Source: CAD feature listing. Evaluate the final solid. Frame: model axes, mm. A direction names the side the tool comes from. Round coordinates to 2 decimals unless told otherwise and drop trailing zeros. Write each loop counter-clockwise with the first axis right and the second up, starting at its lowest first coordinate (ties: lowest second). Pieces come first, ordered by that corner, then holes. Notation, with made-up numbers: M -11,41 L 41,41 A25 cw 41,57 Z; hole C 81,80.5 d9. An arc over 180 degrees is marked long. Answer in a Markdown table with one row per item.
Autodesk Inventor part; units mm, degrees
ref_plane "Work Plane1" through (1.525, 0, 0) normal (0, 0, 1) x (1, 0, 0)
ref_plane "YZ Plane" through (0, 0, 0) normal (1, 0, 0) x (0, 1, 0)
ref_plane "XZ Plane" through (0, 0, 0) normal (0, 1, 0) x (-1, 0, 0)
sketch "草图1" plane through (0, 0, 0) normal (0, 0, 1) x (1, 0, 0)
  line L0 (0, 5.8) -> (0, 4)
  line L1 (1.25, 4) -> (25, 4)
  line L2 (25, 4) -> (25, 0)
  line L3 (25, 0) -> (-0.6001, 0)
  line L4 (-5.7201, 0) -> (30.12, 0)
  line L5 (-0.6001, 0) -> (-0.6001, 5.8)
  line L6 (-0.6001, 5.8) -> (0, 5.8)
  line L7 (1.25, 4) -> (0.4831, 4)
  line L8 (0.4831, 4) -> (0, 4)
  line L9 (0, -1.16) -> (0, 6.96)
  dimension "d0" = 25
  dimension "d1" = 23.75
  dimension "d2" = 8
  dimension "d9" = 0.6001
  dimension "d10" = 11.6
  dimension "d13" = 0.7669
  dimension "d14" = 8
revolve "轴承体" add sketch "草图1" angle 360 about axis through (25, 0, 0) along (-1, 0, 0)
sketch "草图2" plane through (-0.6001, 0, 0) normal (-1, 0, 0) x (0, 0, 1)
  line L0 (0, 7.5056) -> (6.5, 3.7528)
  line L1 (6.5, 3.7528) -> (6.5, -3.7528)
  line L2 (6.5, -3.7528) -> (0, -7.5056)
  line L3 (0, -7.5056) -> (-6.5, -3.7528)
  line L4 (-6.5, -3.7528) -> (-6.5, 3.7528)
  line L5 (-6.5, 3.7528) -> (0, 7.5056)
  point P0 (0, 0)
  point P1 (0, 0)
  dimension "d11" = 13
extrude "头" add sketch "草图2" along normal blind 4.7
sketch "草图4" plane through (0, 0, 0) normal (0, 0, 1) x (1, 0, 0)
  line L0 (-5.3001, 6.5) -> (-5.3001, 7.5056)
  line L1 (-5.3001, 7.5056) -> (-4.7195, 7.5056)
  line L2 (-4.7195, 7.5056) -> (-5.3001, 6.5)
  line L3 (-6.2401, 0) -> (0.3399, 0)
  line L4 (-0.6001, 7.5056) -> (-5.3001, 7.5056)
  line L5 (-5.3001, 3.7528) -> (-5.3001, 7.5056)
  dimension "d5" = 30
  dimension "d19" = 13
revolve "倒角1" cut sketch "草图4" angle 360 about axis through (-10, 0, 0) along (1, 0, 0)
thread "螺纹"
chamfer "倒角2" distance 0.7668 distance2 0.7669 1 edges at (25, -4, 0) measured on face at (25, 0.998, -0.8842)
ref_plane "Work Plane1" through (1.525, 0, 0) normal (0, 0, 1) x (1, 0, 0)
equation "\"d11\" = SW"
equation "\"d3\" = KOH - SD"
equation "\"d15\" = GEL"
equation "\"d6\" = -0.5 * SPD + 0.5 * GD"
equation "\"d0\" = NLG"
equation "\"d1\" = GEL"
equation "\"d2\" = GD"
equation "\"d10\" = SD2"
equation "\"d14\" = BDM"
equation "\"d5\" = ANG1"
equation "\"d19\" = SW0"
equation "\"NLG\" = 25"
equation "\"GD\" = NND"
equation "\"BDM\" = NND"
equation "\"KOH\" = 5.3"
equation "\"GEL\" = 23.75"
equation "\"SW\" = 13"
equation "\"SW0\" = SW"
equation "\"SPD\" = NND - 1.2269 * PTC"
equation "\"SD2\" = SDH"
equation "\"SD\" = WFT"
equation "\"ANG1\" = 30deg"
equation "\"GAL\" = 0.61345 * PTC"
equation "\"GUL\" = 0.61345 * PTC"
equation "\"RR\" = 0.4"
equation "\"WFT\" = 0.6"
equation "\"GD1\" = THREADDIA - 1.2269 * PTC"
equation "\"THREADDIA\" = 8"
equation "\"SDH\" = 11.6"
equation "\"TOA\" = 30deg"
equation "\"FAWI\" = 45deg"
equation "\"PTC\" = 1.25"
equation "\"NND\" = 8"
equation "\"E0\" = 1.155 * SW"
properties part number "螺栓 GB/T 5783 M8 x 25" material "钢，软"
Q1. Section A-A (x = 20.5). Return loops of the section in (y, z).
Solutions:
| item | result |
|---|---|
| outline | C 0,0 d8 |
Q2. Material intervals for probe 1 along Y at (x, z) = (15, 0); probe 2 along X at (y, z) = (2, -4.5); probe 3 along X at (y, z) = (3, -5.5), sorted ascending.
Solutions:
| item | result |
|---|---|
| probe 1 | y = -4 to 4 |
| probe 2 | x = -5.3 to 0 |
| probe 3 | x = -5.3 to -0.6 |
Q3. Access query for faces 1 (the flat face through (-0.6, -6, -2)), 2 (the flat face through (-3, 0, 6.5)). Directions: +Z, -Z, +X, -X, +Y, -Y. A direction counts if a zero-diameter tool reaches every point of the face in a straight line with its end or side. Return the directions, or none.
Solutions:
| item | result |
|---|---|
| face 1 | +X |
| face 2 | +Z, +X, -X, +Y, -Y |
Q4. Contact query for flat-ended pins moving along their axis: pin 1 Ø5 at (x, z) = (11, 2.5) entering from +Y; pin 2 Ø3 at (x, y) = (7.5, 4) entering from -Z; pin 3 Ø6 at (x, y) = (14.5, 3) entering from -Z. Output: stop coordinate, or through.
Solutions:
| item | result |
|---|---|
| pin 1 | stops at y = 4 |
| pin 2 | stops at z = -3.12 |
| pin 3 | stops at z = -4 |
